Work out the finished part from the listing and answer in its coordinate system (mm). A direction names the side the tool comes from. Coordinates: 2 decimals unless noted, no trailing zeros. Order: outer loops, then holes, each group sorted by start corner. A loop starts at its lowest first (then second) coordinate and runs counter-clockwise, first axis right, second up. Notation, with made-up numbers: (62, -14.75) -> (80, -14.75) arc R22 ccw to (80, -5.75) -> close; hole circle Ø6 at (3.5, 13.25). An arc over 180 degrees is marked (long way). Use one line per item in the form item = value.
from build123d import *

# Parameters (mm, degrees)
MAIN_DEPTH         = 20
SKETCH3_R          = 2.25
SCREW_HOLE_DEPTH   = 459.547512827
SKETCH4_R          = 2.75
SCREW_HOLE_2_DEPTH = 461.247257207
SCREW_CUT_R        = 5
SCREWCUT_DEPTH     = 16
CUT_EXTRUDE7_START = -5
SKETCH7_R          = 4
CUT_EXTRUDE7_DEPTH = 5
RIB3_REACH         = 57.989
SKETCH8_WALL_W     = 136.182475206
SKETCH8_WALL_H     = 5
RIB4_START         = -5
RIB4_DEPTH         = 5
CHAMFER1_SIZE      = 1


# Read off the part's stored shape, not the designer's step: Rib4
with BuildPart() as part:
    # Sketch2 → main (new body)
    with BuildSketch(Plane(origin=(0, -457.638253618, -1.412254138), x_dir=(1, 0, 0), z_dir=(0, 1, 0))):
        Polygon((25.505676484, -2.181428465), (32.505676484, -2.181428465), (32.505676484, -20.181428465), (45.505676484, -20.181428465), (45.505676484, -27.181428465), (25.505676484, -27.181428465), align=None)
    extrude(amount=MAIN_DEPTH)

    # Sketch3 → screw_hole (cut, through all)
    with BuildSketch(Plane(origin=(32.505676484, 0, 0), x_dir=(0, 0, -1), z_dir=(1, 0, 0))):
        with Locations((-6.769174326, -447.638253618)):
            Circle(SKETCH3_R)
    extrude(amount=-SCREW_HOLE_DEPTH, mode=Mode.SUBTRACT)

    # Sketch4 → screw_hole_2 (cut, through all)
    with BuildSketch(Plane(origin=(0, 0, 18.769174326), x_dir=(-1, 0, 0), z_dir=(0, 0, -1))):
        with Locations((-35.505676484, -447.638253618)):
            Circle(SKETCH4_R)
    extrude(amount=-SCREW_HOLE_2_DEPTH, mode=Mode.SUBTRACT)

    # screw_cut → screwcut (cut)
    with BuildSketch(Plane(origin=(0, 0, 18.769174326), x_dir=(-1, 0, 0), z_dir=(0, 0, -1))):
        with Locations((-35.505676484, -447.638253618)):
            Circle(SCREW_CUT_R)
    extrude(amount=SCREWCUT_DEPTH, mode=Mode.SUBTRACT)

    # Sketch7 → Cut-Extrude7 (cut)
    with BuildSketch(Plane.ZY.offset(-25.505676484).offset(CUT_EXTRUDE7_START)):
        with Locations((6.769174326, -447.638253618)):
            Circle(SKETCH7_R)
    extrude(amount=-CUT_EXTRUDE7_DEPTH, mode=Mode.SUBTRACT)

    # Sketch8 wall → Rib3 (add, up to next)
    with BuildSketch(Plane(origin=(39.005676484, -457.638253618, 9.769174326), x_dir=(0.585490553844, 0, 0.8106792284), z_dir=(-0.8106792284, 0, 0.585490553844)), mode=Mode.PRIVATE) as rib3_sk1:
        with Locations((0, 2.5)):
            Rectangle(SKETCH8_WALL_W, SKETCH8_WALL_H)
    rib3_tool1 = extrude(rib3_sk1.sketch, amount=RIB3_REACH, mode=Mode.PRIVATE) - part.part
    add(rib3_tool1.solids().sort_by_distance((39.005676484, -457.638253618, 9.769174326))[0])

    # Rib4 outline → Rib4 (add)
    with BuildSketch(Plane(origin=(0, -437.638253618, 0), x_dir=(1, 0, 0), z_dir=(0, 1, 0)).offset(RIB4_START)):
        Polygon((45.505676484, -18.769174326), (32.505676484, -0.769174326), (32.505676484, -18.769174326), align=None)
    extrude(amount=RIB4_DEPTH)

    # Chamfer1
    chamfer1_edges = [part.edges().sort_by_distance(p)[0] for p in [
        (45.505676484, -437.638253618, 22.269174326),
        (39.005676484, -452.638253618, 9.769174326),
        (39.005676484, -457.638253618, 9.769174326),
        (45.505676484, -457.638253618, 22.269174326),
        (39.005676484, -442.638253618, 9.769174326),
        (39.005676484, -437.638253618, 9.769174326),
    ]]
    chamfer(chamfer1_edges, length=CHAMFER1_SIZE)


solid = part.part
(1) Each of these flat-tipped pins is pushed along its axis until it touches: P1, Ø4, axis at y = -447.64, z = 6.77, coming from the +X side; P2, Ø6.5, axis at y = -447, z = 8, coming from the +X side; P3, Ø6, axis at y = -445, z = 12.5, coming from the +X side; P4, Ø6, axis at x = 40.5, y = -450.5, coming from the -Z side. Where does it stop, or does it pass through?
Data:
P1 = through
P2 = 32.36
P3 = 41.12
P4 = 10.6
(2) Section C-C on z = 22.5 is taken. Write down the section's boundary in (x, y).
Data:
outline = (25.51, -457.64) -> (44.51, -457.64) -> (45.51, -456.64) -> (45.51, -438.64) -> (44.51, -437.64) -> (25.51, -437.64) -> close; hole circle Ø5.5 at (35.51, -447.64)
(3) Section B-B on x = 37.5 is taken. Write down the section's boundary in (y, z).
Data:
outline = (-457.64, 9.39) -> (-456.64, 7.68) -> (-453.64, 7.68) -> (-452.64, 9.39) -> (-452.64, 18.77) -> (-449.53, 18.77) -> (-449.53, 25.77) -> (-457.64, 25.77) -> close; (-445.74, 18.77) -> (-442.64, 18.77) -> (-442.64, 9.39) -> (-441.64, 7.68) -> (-438.64, 7.68) -> (-437.64, 9.39) -> (-437.64, 25.77) -> (-445.74, 25.77) -> close
(4) Which of the six approach directions +Z, -Z, +X, -X, +Y, -Y give full straight-line access (tool end or side, diameter ignored) to faces 4 (the flat face through (38, -452.638, 14)), 5 (the cylindrical face through (31.7, -450.88, 3.89)), 6 (the flat face through (32, -457.638, 15))?
Data:
face_4 = -Z, +X
face_5 = +X
face_6 = +Z, -Z, +X, -X, -Y
(5) Section D-D on z = 7.75 is taken. Write down the section's boundary in (x, y).
Data:
outline = (25.51, -457.64) -> (36.31, -457.64) -> (37.55, -456.64) -> (37.55, -453.64) -> (36.31, -452.64) -> (32.51, -452.64) -> (32.51, -451.64) arc R5 cw to (32.35, -451.52) -> (30.51, -451.52) -> (30.51, -449.66) -> (25.51, -449.66) -> close; (25.51, -445.61) -> (30.51, -445.61) -> (30.51, -443.76) -> (32.35, -443.76) arc R5 cw to (32.51, -443.64) -> (32.51, -442.64) -> (36.31, -442.64) -> (37.55, -441.64) -> (37.55, -438.64) -> (36.31, -437.64) -> (25.51, -437.64) -> close
(6) Straight lines are drawn through the part: line 1 along Z through (x, y) = (41.5, -448.75); line 2 along X through (y, z) = (-451.25, 7.25); line 3 along Y through (x, z) = (31.75, 9.5). For each, find the intervals that lie inside material, in ascending order.
Data:
line_1 = 18.77 to 25.77
line_2 = 25.51 to 30.51
line_3 = -457.64 to -450.94, -444.34 to -437.64
(7) Section A-A on y = -447.25 is taken. Count the separate pieces of the cut face and the enclosed holes in it, plus the area to 3 significant figures.
Data:
separate_pieces = 3
enclosed_holes = 0
area = 174 mm²
(8) The mould has two halves that part along Y. Classify faces 1 (the cylindrical face through (30.506, -447.703, 14.187)), 2 (the flat face through (39.1, -440.2, 9.9)), 3 (the flat face through (38.477, -438.131, 9.903)): released by +Y, released by -Y, zero draft, split by the parting line, or undercut.
Data:
face_1 = undercut
face_2 = zero draft
face_3 = released by +Y
